Input: part model. Units: mm. Frame: model coordinates. Face numbers are marked on the shaded views. Give positions to 0.01 mm unless a question says otherwise; leave off trailing zeros. Loops run counter-clockwise (first coordinate to the right, second up) from the corner with the lowest first, then second, coordinate; pieces in that order, holes last.
Autodesk Inventor part; units mm, degrees
ref_plane "YZ Plane" through (0, 0, 0) normal (1, 0, 0) x (0, 1, 0)
ref_plane "XZ Plane" through (0, 0, 0) normal (0, 1, 0) x (-1, 0, 0)
ref_plane "XY Plane" through (0, 0, 0) normal (0, 0, 1) x (1, 0, 0)
sketch "Эскиз1" plane through (0, 0, 0) normal (0, 1, 0) x (-1, 0, 0)
  circle A0 centre (0, 0) radius 2.5
  circle A1 centre (0, -72.634) radius 2.5
  circle A2 centre (-41.385, -72.634) radius 2.5
  circle A3 centre (-41.385, 0) radius 2.5
  dimension "d1" = 5
  dimension "d3" = 5
  dimension "d5" = 5
  dimension "d7" = 5
extrude "Выдавливание1" add sketch "Эскиз1" against normal blind 4.5
sketch "Эскиз3" plane through (0, 0, 0) normal (0, 1, 0) x (1, 0, 0)
  line L0 (-4.5666, 0.8672) -> (-4.5666, 71.6657)
  line L1 (0.9251, 77.1637) -> (40.5431, 77.1677)
  line L2 (46.0198, 71.7001) -> (46.0348, 0.8657)
  line L3 (40.5334, -4.6343) -> (0.9348, -4.6343)
  arc A0 (-4.5666, 0.8672) -> (0.9348, -4.6343) centre (0.9348, 0.8672) ccw
  arc A1 (46.0198, 71.7001) -> (40.5431, 77.1677) centre (40.551, 71.699) ccw
  arc A2 (40.5334, -4.6343) -> (46.0348, 0.8657) centre (40.5319, 0.8687) ccw
  line L4 (35.1515, 48.9499) -> (35.1515, 54.3499)
  line L5 (35.1515, 54.6499) -> (35.1515, 48.6499)
  line L6 (35.4515, 54.6499) -> (40.8515, 54.6499)
  line L7 (41.1515, 54.6499) -> (35.1515, 54.6499)
  line L8 (40.8515, 48.6499) -> (35.4515, 48.6499)
  line L9 (41.1515, 54.3499) -> (41.1515, 48.9499)
  line L10 (41.1515, 48.6499) -> (41.1515, 54.6499)
  line L11 (35.1515, 48.6499) -> (41.1515, 48.6499)
  arc A3 (0.9251, 77.1637) -> (-4.5666, 71.6657) centre (1.3393, 71.2583) ccw
extrude "Выдавливание2" add sketch "Эскиз3" against normal blind 2 from surface at -4.5
sketch "Эскиз4" plane through (0.9348, -4.5, 4.6343) normal (0, 1, 0) x (1, 0, 0)
  line L0 (-5.5015, 5.5015) -> (-5.5015, 76.3)
  arc A0 (-4.2015, 5.5015) -> (0, 1.3) centre (0, 5.5015) ccw
  line L1 (45.085, 76.3344) -> (45.1, 5.5)
  line L2 (-0.0097, 81.798) -> (39.6083, 81.802)
  arc A1 (-0.0097, 80.5111) -> (-4.2035, 76.3214) centre (-0.0118, 76.3194) ccw
  arc A2 (43.785, 76.3344) -> (39.6083, 80.5111) centre (39.6083, 76.3344) ccw
  arc A3 (39.5985, 1.3) -> (43.785, 5.5) centre (39.585, 5.5) ccw
  line L3 (0, 1.3) -> (39.5985, 1.3)
  line L4 (43.785, 5.5) -> (43.785, 76.3344)
  line L5 (39.6083, 80.5111) -> (-0.0097, 80.5111)
  arc A4 (-5.5015, 5.5015) -> (0, 0) centre (0, 5.5015) ccw
  arc A5 (-0.0097, 81.798) -> (-5.5015, 76.3) centre (0.4044, 75.8926) ccw
  line L6 (-0.0097, 81.798) -> (39.6083, 81.802)
  arc A6 (45.085, 76.3344) -> (39.6083, 81.802) centre (39.6162, 76.3332) ccw
  arc A7 (39.5985, 0) -> (45.1, 5.5) centre (39.5971, 5.5029) ccw
  line L7 (39.5985, 0) -> (0, 0)
  arc A8 (-5.5015, 5.5015) -> (0, 0) centre (0, 5.5015) ccw
  arc A9 (-0.0097, 81.798) -> (-5.5015, 76.3) centre (0.4044, 75.8926) ccw
  arc A10 (45.085, 76.3344) -> (39.6083, 81.802) centre (39.6162, 76.3332) ccw
  arc A11 (45.085, 76.3344) -> (39.6083, 81.802) centre (39.6088, 76.3258) ccw
  arc A12 (39.5985, 0) -> (45.1, 5.5) centre (39.5971, 5.5029) ccw
  line L8 (-5.5015, 5.5015) -> (-5.5015, 76.3)
  line L9 (-0.0097, 81.798) -> (39.6083, 81.802)
  line L10 (45.085, 76.3344) -> (45.1, 5.5082)
  line L11 (39.5985, 0) -> (0, 0)
  line L12 (-4.2015, 5.5015) -> (-4.2035, 76.3214)
  circle A13 centre (40.4502, 77.2683) radius 1.5
  point P0 (-0.9348, 4.6343)
extrude "Выдавливание3" add sketch "Эскиз4" along normal blind 6 contours L0 A5 L2 A11 L1 A7 L7 A4 | A6 A11
sketch "Эскиз5" plane through (-4.5666, -6.5, -71.6657) normal (-1, 0, 0) x (0, 0, 1)
  line L0 (-5.498, 0) -> (0, 0)
  line L1 (55.3, 7) -> (55.3, 3.5)
  line L2 (-0.0344, 8) -> (70.8, 8)
  line L3 (76.3, 0) -> (76.3, 8)
  line L4 (46.8, 7) -> (46.8, 3.5)
  line L5 (46.8, 3.5) -> (55.3, 3.5)
  line L6 (-0.0344, 0) -> (70.8, 0)
  line L7 (46.8, 7) -> (55.3, 7)
  line L8 (74.1657, 6.5) -> (69.1657, 6.5)
  point P0 (71.6657, 6.5)
  point P1 (57.3, 6.5)
  dimension "d24" = 21
  dimension "d25" = 8.5
  dimension "d26" = 3.5
extrude "Выдавливание4" cut sketch "Эскиз5" against normal blind 6
properties part number "Основание" material "Каучук, силиконовый"
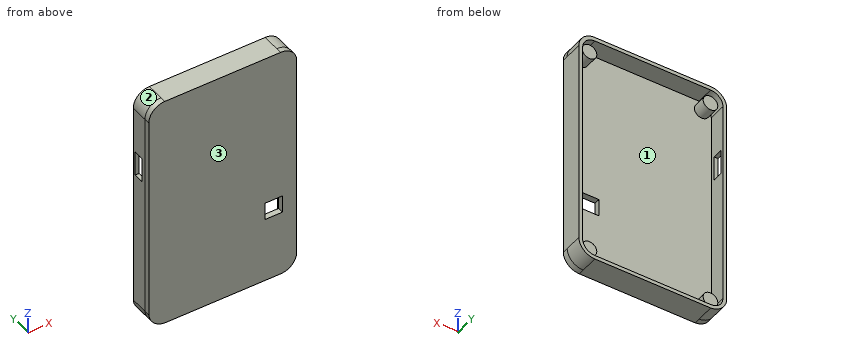
(1) Cut plane B-B (x = 11). Return the cut outline in (y, z).
Values follow:
outline: (-6.5, -77.16) - (1.5, -77.16) - (1.5, -75.88) - (-4.5, -75.88) - (-4.5, 3.33) - (1.5, 3.33) - (1.5, 4.63) - (-6.5, 4.63) - close
(2) Cut plane D-D (z = 0). Return the cut outline in (x, y) (3 decimals), and give its area (3 significant figures).
Values follow:
outline: (-4.498, -6.5) - (45.966, -6.5) - (45.966, 1.5) - (44.63, 1.5) - (44.63, -4.5) - (43.885, -4.5) - (43.885, 0) - (38.885, 0) - (38.885, -4.5) - (2.5, -4.5) - (2.5, 0) - (-2.5, 0) - (-2.5, -4.5) - (-3.176, -4.5) - (-3.176, 1.5) - (-4.498, 1.5) - close
area: 162 mm2
(3) Cut plane C-C (z = -49.5). Return the cut outline in (x, y), and give its area (3 significant figures).
Values follow:
outline: (-4.57, -6.5) - (35.15, -6.5) - (35.15, -4.5) - (-3.27, -4.5) - (-3.27, 1.5) - (-4.57, 1.5) - close; (41.15, -6.5) - (46.02, -6.5) - (46.02, 1.5) - (44.72, 1.5) - (44.72, -4.5) - (41.15, -4.5) - close
area: 105 mm2
(4) Ray query, probe 1 along X at (y, z) = (-1.5, -12); probe 2 along Z at (x, y) = (36.5, -1.5); probe 3 along X at (y, z) = (-3, 1). Return the intervals inside material, ascending.
Values follow:
probe 1: x = -4.57 to -3.27, 44.72 to 46.03
probe 2: z = -77.17 to -75.88, 3.33 to 4.63
probe 3: x = -4.24 to -2.83, -2.29 to 2.29, 39.09 to 43.68, 44.28 to 45.71
(5) Mould query, pull axis Z, two halves, no side actions, for the marked faces 1, 2 and 3. Classes: +Z half, -Z half, draft (parallel to the pull), parting line (faces both ways), or undercut.
Values follow:
face 1: undercut
face 2: +Z half
face 3: draft
(6) Cut plane A-A (y = -1.25). Return the cut outline in (x, z) (1 decimal).
Values follow:
outline: (-4.6, -71.7) arc R5.9 ccw to (0.9, -77.2) - (40.5, -77.2) arc R5.5 ccw to (46, -71.7) - (46, -0.9) arc R5.5 ccw to (40.5, 4.6) - (0.9, 4.6) arc R5.5 ccw to (-4.6, -0.9) - (-4.6, -16.4) - (-3.3, -16.4) - (-3.3, -0.9) arc R4.2 cw to (0.9, 3.3) - (40.5, 3.3) arc R4.2 cw to (44.7, -0.9) - (44.7, -71.7) arc R4.2 cw to (40.5, -75.9) - (0.9, -75.9) arc R4.2 cw to (-3.3, -71.7) - (-3.3, -24.9) - (-4.6, -24.9) - close; circle Ø5 at (0, -72.6); circle Ø5 at (0, 0); circle Ø5 at (41.4, -72.6); circle Ø5 at (41.4, 0)
(7) Pin query (flat end, axial travel): pin 1 Ø14.5 at (x, z) = (32, -46.5) entering from +Y; pin 2 Ø4 at (y, z) = (-2.5, -20.5) entering from +X; pin 3 Ø1.5 at (x, y) = (8, 0.5) entering from -Z. Return the tip coordinate at first contact, or that it passes through.
Values follow:
pin 1: stops at y = -4.5
pin 2: stops at x = 46.03
pin 3: stops at z = -77.16
